For this review, take the finished solid that the model builds, in its own axes (mm). Face numbers are marked on the shaded views. Coordinates: 2 decimals unless noted, no trailing zeros. Loops run counter-clockwise (first coordinate to the right, second up) from the corner with the lowest first, then second, coordinate; pieces in that order, holes last. Notation, with made-up numbers: M 34.5,-20 L 49.5,-20 A20 ccw 49.5,-6 Z; hole C -27,18 d1. An arc over 180 degrees is marked long. Use one line per item in the form item = value.
```python
from build123d import *

# Parameters (mm, degrees)
SKETCH2_W                                       = 84.5
SKETCH2_H                                       = 58.5
BOSS_EXTRUDE1_DEPTH                             = 0.5
BOSS_EXTRUDE2_DEPTH                             = 5
BOSS_EXTRUDE2_DEPTH_BACK                        = 3
SKETCH3_R                                       = 3.5
BOSS_EXTRUDE3_DEPTH                             = 5
BOSS_EXTRUDE3_DEPTH_BACK                        = 3
SKETCH5_R                                       = 3.5
BOSS_EXTRUDE4_DEPTH                             = 5
BOSS_EXTRUDE4_DEPTH_BACK                        = 3
SKETCH6_R                                       = 3.5
BOSS_EXTRUDE5_DEPTH                             = 5
BOSS_EXTRUDE5_DEPTH_BACK                        = 3
SKETCH7_R                                       = 3.5
CSK_FOR_M3_FLAT_HEAD_MACHINE_SCREW1_D           = 3.2
CSK_FOR_M3_FLAT_HEAD_MACHINE_SCREW1_DEPTH       = 13.03862301
CSK_FOR_M3_FLAT_HEAD_MACHINE_SCREW1_CSINK_D     = 6.3
CSK_FOR_M3_FLAT_HEAD_MACHINE_SCREW1_CSINK_ANGLE = 90
CSK_FOR_M3_FLAT_HEAD_MACHINE_SCREW1_TIP         = 0.96137699
CSK_FOR_M3_FLAT_HEAD_MACHINE_SCREW2_D           = 3.2
CSK_FOR_M3_FLAT_HEAD_MACHINE_SCREW2_DEPTH       = 13.03862301
CSK_FOR_M3_FLAT_HEAD_MACHINE_SCREW2_CSINK_D     = 6.3
CSK_FOR_M3_FLAT_HEAD_MACHINE_SCREW2_CSINK_ANGLE = 90
CSK_FOR_M3_FLAT_HEAD_MACHINE_SCREW2_TIP         = 0.96137699
CSK_FOR_M3_FLAT_HEAD_MACHINE_SCREW3_D           = 3.2
CSK_FOR_M3_FLAT_HEAD_MACHINE_SCREW3_DEPTH       = 13.03862301
CSK_FOR_M3_FLAT_HEAD_MACHINE_SCREW3_CSINK_D     = 6.3
CSK_FOR_M3_FLAT_HEAD_MACHINE_SCREW3_CSINK_ANGLE = 90
CSK_FOR_M3_FLAT_HEAD_MACHINE_SCREW3_TIP         = 0.96137699
CSK_FOR_M3_FLAT_HEAD_MACHINE_SCREW4_D           = 3.2
CSK_FOR_M3_FLAT_HEAD_MACHINE_SCREW4_DEPTH       = 13.03862301
CSK_FOR_M3_FLAT_HEAD_MACHINE_SCREW4_CSINK_D     = 6.3
CSK_FOR_M3_FLAT_HEAD_MACHINE_SCREW4_CSINK_ANGLE = 90
CSK_FOR_M3_FLAT_HEAD_MACHINE_SCREW4_TIP         = 0.96137699


with BuildPart() as part:
    # Sketch2 → Boss-Extrude1 (new body)
    with BuildSketch(Plane(origin=(0, 0, 0), x_dir=(1, 0, 0), z_dir=(0, 1, 0))):
        with Locations((-42.25, -29.25)):
            Rectangle(SKETCH2_W, SKETCH2_H)
    extrude(amount=BOSS_EXTRUDE1_DEPTH)

    # Sketch3 → Boss-Extrude2 (add, two sides: drawn at the far end of the back side and taken through both)
    with BuildSketch(Plane(origin=(0, 0.5, 0), x_dir=(1, 0, 0), z_dir=(0, 1, 0)).offset(-BOSS_EXTRUDE2_DEPTH_BACK)):
        with Locations(Location((-84.5, 0, 0), (0, 0, 270))):
            Circle(SKETCH3_R)
    extrude(amount=BOSS_EXTRUDE2_DEPTH + BOSS_EXTRUDE2_DEPTH_BACK)

    # Sketch5 → Boss-Extrude3 (add, two sides: drawn at the far end of the back side and taken through both)
    with BuildSketch(Plane(origin=(0, 0.5, 0), x_dir=(1, 0, 0), z_dir=(0, 1, 0)).offset(-BOSS_EXTRUDE3_DEPTH_BACK)):
        with Locations(Location((-84.5, -58.5, 0), (0, 0, 270))):
            Circle(SKETCH5_R)
    extrude(amount=BOSS_EXTRUDE3_DEPTH + BOSS_EXTRUDE3_DEPTH_BACK)

    # Sketch6 → Boss-Extrude4 (add, two sides: drawn at the far end of the back side and taken through both)
    with BuildSketch(Plane(origin=(0, 0.5, 0), x_dir=(1, 0, 0), z_dir=(0, 1, 0)).offset(-BOSS_EXTRUDE4_DEPTH_BACK)):
        with Locations(Location((0, -58.5, 0), (0, 0, 270))):
            Circle(SKETCH6_R)
    extrude(amount=BOSS_EXTRUDE4_DEPTH + BOSS_EXTRUDE4_DEPTH_BACK)

    # Sketch7 → Boss-Extrude5 (add, two sides: drawn at the far end of the back side and taken through both)
    with BuildSketch(Plane(origin=(0, 0.5, 0), x_dir=(1, 0, 0), z_dir=(0, 1, 0)).offset(-BOSS_EXTRUDE5_DEPTH_BACK)):
        with Locations(Location((0, 0, 0), (0, 0, 270))):
            Circle(SKETCH7_R)
    extrude(amount=BOSS_EXTRUDE5_DEPTH + BOSS_EXTRUDE5_DEPTH_BACK)

    # CSK for M3 Flat Head Machine Screw1
    with Locations(Plane(origin=(0, 5.5, 0), x_dir=(1, 0, 0), z_dir=(0, 1, 0))):
        with Locations((-84.5, 0)):
            CounterSinkHole(CSK_FOR_M3_FLAT_HEAD_MACHINE_SCREW1_D / 2, CSK_FOR_M3_FLAT_HEAD_MACHINE_SCREW1_CSINK_D / 2, depth=CSK_FOR_M3_FLAT_HEAD_MACHINE_SCREW1_DEPTH, counter_sink_angle=CSK_FOR_M3_FLAT_HEAD_MACHINE_SCREW1_CSINK_ANGLE)
            with Locations((0, 0, -(CSK_FOR_M3_FLAT_HEAD_MACHINE_SCREW1_DEPTH + CSK_FOR_M3_FLAT_HEAD_MACHINE_SCREW1_TIP / 2))):  # 118° drill point
                Cone(0, CSK_FOR_M3_FLAT_HEAD_MACHINE_SCREW1_D / 2, CSK_FOR_M3_FLAT_HEAD_MACHINE_SCREW1_TIP, mode=Mode.SUBTRACT)

    # CSK for M3 Flat Head Machine Screw2
    with Locations(Plane(origin=(0, 5.5, 0), x_dir=(1, 0, 0), z_dir=(0, 1, 0))):
        with Locations((-84.5, -58.5)):
            CounterSinkHole(CSK_FOR_M3_FLAT_HEAD_MACHINE_SCREW2_D / 2, CSK_FOR_M3_FLAT_HEAD_MACHINE_SCREW2_CSINK_D / 2, depth=CSK_FOR_M3_FLAT_HEAD_MACHINE_SCREW2_DEPTH, counter_sink_angle=CSK_FOR_M3_FLAT_HEAD_MACHINE_SCREW2_CSINK_ANGLE)
            with Locations((0, 0, -(CSK_FOR_M3_FLAT_HEAD_MACHINE_SCREW2_DEPTH + CSK_FOR_M3_FLAT_HEAD_MACHINE_SCREW2_TIP / 2))):  # 118° drill point
                Cone(0, CSK_FOR_M3_FLAT_HEAD_MACHINE_SCREW2_D / 2, CSK_FOR_M3_FLAT_HEAD_MACHINE_SCREW2_TIP, mode=Mode.SUBTRACT)

    # CSK for M3 Flat Head Machine Screw3
    with Locations(Plane(origin=(0, 5.5, 0), x_dir=(1, 0, 0), z_dir=(0, 1, 0))):
        with Locations((0, 0)):
            CounterSinkHole(CSK_FOR_M3_FLAT_HEAD_MACHINE_SCREW3_D / 2, CSK_FOR_M3_FLAT_HEAD_MACHINE_SCREW3_CSINK_D / 2, depth=CSK_FOR_M3_FLAT_HEAD_MACHINE_SCREW3_DEPTH, counter_sink_angle=CSK_FOR_M3_FLAT_HEAD_MACHINE_SCREW3_CSINK_ANGLE)
            with Locations((0, 0, -(CSK_FOR_M3_FLAT_HEAD_MACHINE_SCREW3_DEPTH + CSK_FOR_M3_FLAT_HEAD_MACHINE_SCREW3_TIP / 2))):  # 118° drill point
                Cone(0, CSK_FOR_M3_FLAT_HEAD_MACHINE_SCREW3_D / 2, CSK_FOR_M3_FLAT_HEAD_MACHINE_SCREW3_TIP, mode=Mode.SUBTRACT)

    # CSK for M3 Flat Head Machine Screw4
    with Locations(Plane(origin=(0, 5.5, 0), x_dir=(1, 0, 0), z_dir=(0, 1, 0))):
        with Locations((0, -58.5)):
            CounterSinkHole(CSK_FOR_M3_FLAT_HEAD_MACHINE_SCREW4_D / 2, CSK_FOR_M3_FLAT_HEAD_MACHINE_SCREW4_CSINK_D / 2, depth=CSK_FOR_M3_FLAT_HEAD_MACHINE_SCREW4_DEPTH, counter_sink_angle=CSK_FOR_M3_FLAT_HEAD_MACHINE_SCREW4_CSINK_ANGLE)
            with Locations((0, 0, -(CSK_FOR_M3_FLAT_HEAD_MACHINE_SCREW4_DEPTH + CSK_FOR_M3_FLAT_HEAD_MACHINE_SCREW4_TIP / 2))):  # 118° drill point
                Cone(0, CSK_FOR_M3_FLAT_HEAD_MACHINE_SCREW4_D / 2, CSK_FOR_M3_FLAT_HEAD_MACHINE_SCREW4_TIP, mode=Mode.SUBTRACT)


solid = part.part
```
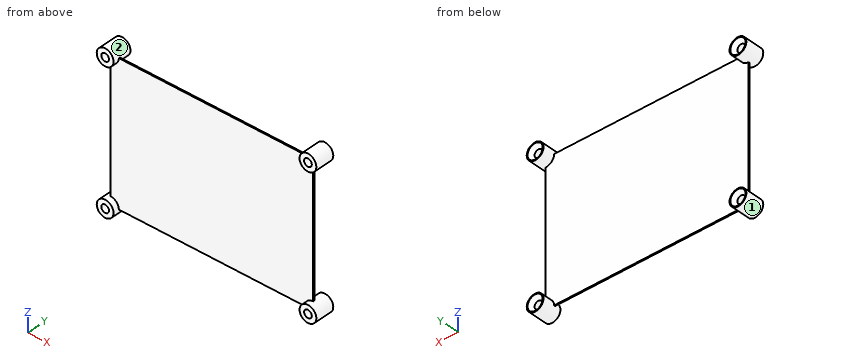
1. For pin 1 Ø2 at (x, z) = (-30.5, 53) entering from +Y; pin 2 Ø0.6 at (y, z) = (0, 32) entering from -X; pin 3 Ø0.6 at (x, y) = (-58.5, 0) entering from -Z, all flat-tipped, find the tip position at first contact; note any pin that passes through.
Computed values:
pin_1 = 0.5
pin_2 = -84.5
pin_3 = 0
2. Wall thickness on line 1 along Y through (x, z) = (-16, 42); line 2 along Z through (x, y) = (-2, 2.5): over which ranges is each line inside the solid? List them lowest first. Write a range as from..to.
Computed values:
line_1 = 0..0.5
line_2 = -2.87..2.87, 55.63..61.37
3. Consider section A-A on x = -76. Write out the cut boundary in (y, z), plus the area to 4 significant figures.
Computed values:
outline = M 0,0 L 0.5,0 L 0.5,58.5 L 0,58.5 Z
area = 29.25 mm2
4. Consider section B-B on z = 38.5. Write out the cut boundary in (x, y), plus the area to 4 significant figures.
Computed values:
outline = M -84.5,0 L 0,0 L 0,0.5 L -84.5,0.5 Z
area = 42.25 mm2
5. Draft analysis for pull direction Z (two halves, no side actions). For the marked faces 1 and 2, state which applies: +Z half, -Z half, draft (parallel to the pull), parting line (faces both ways), or undercut.
Computed values:
face_1 = undercut
face_2 = undercut
